Verification items for the finished model (mm, model axes). A direction names the side the tool comes from. Coordinates: 2 decimals unless noted, no trailing zeros. Write each loop counter-clockwise with the first axis right and the second up, starting at its lowest first coordinate (ties: lowest second). Pieces come first, ordered by that corner, then holes.
```python
from build123d import *

# Parameters (mm, degrees)
F1_DEPTH = 13
F2_W     = 1.5
F2_H     = 3


with BuildPart() as f1:
    # F0 (on Top) → F1 (new body)
    with BuildSketch(Plane.XY):
        with BuildLine():
            Line((21.15, 11.15), (4.75, 27.55))
            ThreePointArc((4.75, 27.55), (0, 22.8), (-4.75, 27.55))
            Line((-4.75, 27.55), (-21.15, 11.15))
            Line((-21.15, 11.15), (-10, 0))
            Line((-10, 0), (0, 0))
            Line((0, 0), (10, 0))
            Line((10, 0), (21.15, 11.15))
        make_face()
    extrude(amount=F1_DEPTH)

    # F3: sweep along a path in F3_path
    with BuildLine(Plane(origin=(-4.75, 27.55, 13), x_dir=(0, -1, 0), z_dir=(0, 0, -1))) as f3_path:
        ThreePointArc((0, 0), (4.75, -4.75), (0, -9.5))
    # F2 (on face) → F3 (sweep, cut)
    with BuildSketch(Plane(origin=(16.15, 16.15, 0), x_dir=(-0.7071067812, 0.7071067812, 0), z_dir=(0.7071067812, 0.7071067812, 0))):
        with Locations((12.3720346111, 6.5)):
            Rectangle(F2_W, F2_H)
    sweep(path=f3_path.line, mode=Mode.SUBTRACT)


solid = f1.part
```
1. Gauge pin test, flat ends, axial feed: P1, Ø4, axis at y = 22.5, z = 2.5, coming from the -X side; P2, Ø1.5, axis at y = 12, z = 6.5, coming from the +X side; P3, Ø1.5, axis at x = -12.5, z = 7.5, coming from the -Y side. Record the tip position at first contact, or that the pin passes through.
2. Sectioned sample at D-D, the plane y = 10. Record the boundary of the cut face in (x, z).
3. Tool access check on faces 1 (the flat face through (13.1, 19.2, 6.4)), 2 (the flat face through (0, 20, 5)). Record the directions out of +Z, -Z, +X, -X, +Y, -Y that give a thin tool (end or side, any length) a straight path to the whole face; none if there is none.
4. Material ranges on L1, parallel to Z at x = 1, y = 19.25; L2, parallel to X at y = 24.5, z = 0.5; L3, parallel to X at y = 24.75, z = 3, recorded low to high.
5. Sectioned sample at A-A, the plane z = 7.25. Record the boundary of the cut face in (x, y).
6. Draft check along Z on faces 3 (the flat face through (0, 11, 0)), 4 (the flat face through (15, 5, 6)), 5 (the flat face through (0, 11, 13)), 6 (the cylindrical face through (-0.142, 19.005, 6.479)). Enter one of: pulls with the +Z half, pulls with the -Z half, needs draft (parallel to the pull), parting line crosses it, or undercut.
7. Sectioned sample at C-C, the plane z = 1. Record the boundary of the cut face in (x, y).
8. Sectioned sample at B-B, the plane x = 5.5. Record the boundary of the cut face in (y, z), and give its area (3 significant figures).
Outcome:
1. P1: stops at x = -11.8
1. P2: stops at x = 21.05
1. P3: stops at y = 1.75
2. outline: (-20, 0) - (20, 0) - (20, 13) - (-20, 13) - close
3. face 1: +Z, -Z, +X, +Y
3. face 2: none
4. L1: z = 0 to 5, 8 to 13
4. L2: x = -7.8 to -3.64, 3.64 to 7.8
4. L3: x = -7.55 to -3.84, 3.84 to 7.55
5. outline: (-21.15, 11.15) - (-10, 0) - (10, 0) - (21.15, 11.15) - (7.93, 24.37) arc R8.55 cw to (-7.93, 24.37) - close; (-6.87, 25.43) arc R7.19 ccw to (6.87, 25.43) - (4.75, 27.55) arc R4.75 cw to (-4.75, 27.55) - close
6. face 3: pulls with the -Z half
6. face 4: needs draft
6. face 5: pulls with the +Z half
6. face 6: undercut
7. outline: (-21.15, 11.15) - (-10, 0) - (10, 0) - (21.15, 11.15) - (4.75, 27.55) arc R4.75 cw to (-4.75, 27.55) - close
8. outline: (0, 0) - (26.8, 0) - (26.8, 13) - (0, 13) - close; hole (21.01, 5) - (22.92, 5) - (22.92, 8) - (21.01, 8) - close
8. area: 343 mm2
